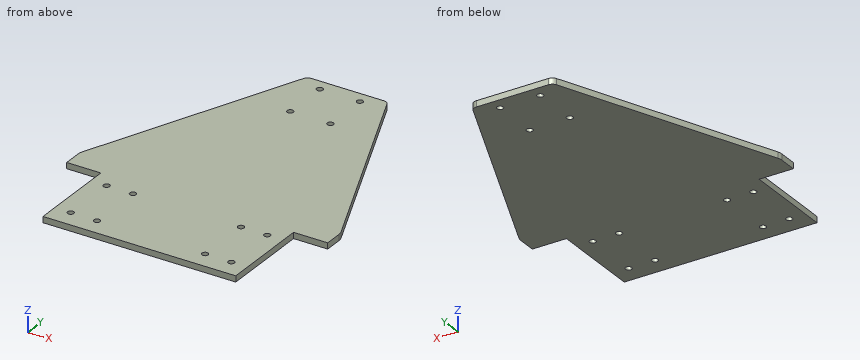
Autodesk Fusion 360 part; units mm, degrees
sketch "Main" plane through (0, 0, 0) normal (0, 0, 1) x (1, 0, 0)
  line L0 (0, 55) -> (45, 162)
  line L1 (45, 162) -> (85, 162)
  line L2 (85, 162) -> (130, 55)
  line L3 (113, 0) -> (17, 0)
  line L4 (65, 0) -> (65, 162) construction
  line L5 (0, 55) -> (0, 45)
  line L6 (0, 45) -> (17, 45)
  line L7 (17, 45) -> (17, 0)
  line L8 (130, 55) -> (130, 45)
  line L9 (130, 45) -> (113, 45)
  line L10 (113, 45) -> (113, 0)
  dimension "d2" = 162
  dimension "d6" = 55
  dimension "d9" = 40
  dimension "d45" = 130
  dimension "d47" = 17
  dimension "d48" = 17
  dimension "d49" = 10
  dimension "d50" = 10
extrude "Extrude1" add sketch "Main" along normal blind 3
sketch "Head Tube Holes" plane through (0, 0, 3) normal (0, 0, 1) x (-1, 0, 0)
  line L0 (-17, 0) -> (-113, 0)
  line L1 (-130, -55) -> (-85, -162)
  line L2 (-85, -162) -> (-45, -162)
  line L3 (-45, -162) -> (0, -55)
  circle A0 centre (-55, -156) radius 1.55
  line L4 (-65, -162) -> (-65, 0) construction
  circle A1 centre (-75, -156) radius 1.55
  circle A2 centre (-55, -133) radius 1.55
  circle A3 centre (-75, -133) radius 1.55
  line L5 (0, -55) -> (0, -45)
  line L6 (0, -45) -> (-17, -45)
  line L7 (-17, -45) -> (-17, 0)
  line L8 (-113, 0) -> (-113, -45)
  line L9 (-113, -45) -> (-130, -45)
  line L10 (-130, -45) -> (-130, -55)
  dimension "d19" = 3.1
  dimension "d20" = 6
  dimension "d21" = 10
  dimension "d24" = -20
  dimension "d25" = 23
extrude "Extrude2" cut sketch "Head Tube Holes" against normal up to surface (3 mm away) contours A0 | A1 | A2 | A3
sketch "Motor Box Holes" plane through (0, 0, 3) normal (0, 0, 1) x (-1, 0, 0)
  circle A0 centre (-75, -156) radius 1.55
  circle A1 centre (-55, -156) radius 1.55
  circle A2 centre (-75, -133) radius 1.55
  circle A3 centre (-55, -133) radius 1.55
  line L0 (-17, 0) -> (-113, 0)
  line L1 (-17, -37) -> (-113, -37) construction
  circle A4 centre (-25, -37) radius 1.55
  circle A5 centre (-38.1, -37) radius 1.55
  circle A6 centre (-25, -9.1) radius 1.55
  circle A7 centre (-38.1, -9.1) radius 1.55
  circle A8 centre (-105, -37) radius 1.55
  circle A9 centre (-91.9, -37) radius 1.55
  circle A10 centre (-105, -9.1) radius 1.55
  circle A11 centre (-91.9, -9.1) radius 1.55
  line L2 (-17, -45) -> (-17, 0)
  line L3 (-113, 0) -> (-113, -45)
  dimension "d30" = 3.1
  dimension "d32" = 37
  dimension "d35" = -13.1
  dimension "d36" = 27.9
  dimension "d37" = 3.1
  dimension "d40" = 13.1
  dimension "d41" = 27.9
  dimension "d53" = 8
  dimension "d54" = 8
extrude "Extrude3" cut sketch "Motor Box Holes" against normal through all contours A4 | A5 | A6 | A7 | A8 | A9 | A10 | A11
fillet "Fillet5" radius 3 2 edges at (45, 162, 1.5) (85, 162, 1.5)
fillet "Fillet6" radius 6 2 edges at (0, 55, 1.5) (130, 55, 1.5)
Work out the finished part from the listing and answer in its coordinate system (mm). Round coordinates to 2 decimals unless told otherwise and drop trailing zeros. Write each loop counter-clockwise with the first axis right and the second up, starting at its lowest first coordinate (ties: lowest second). Pieces come first, ordered by that corner, then holes. Notation, with made-up numbers: (7, 80.5) - (38, 80.5) arc R25 ccw to (38, 115.5) - close; hole circle Ø8 at (70, -31.75). An arc over 180 degrees is marked (long way). Answer in a Markdown table with one row per item. Add a question column.
1. Given pin 1 (3 mm diameter, centred on x = 105, y = 9.1, fed in from +Z); pin 2 (0.9 mm diameter, centred on y = 31, z = 2, fed in from -X); pin 3 (0.9 mm diameter, centred on y = 13.5, z = 2, fed in from +X); pin 4 (1.5 mm diameter, centred on x = 120.5, z = 2, fed in from -Y), each flat-ended and moving along its own axis, determine where each tip first touches the part or whether it passes through.
2. Find the intervals of material crossed by line 1 along Y through (x, z) = (75, 1.85); line 2 along X through (y, z) = (37, 2.05); line 3 along X through (y, z) = (133, 1.35), in increasing order. Write a range as from..to.
3. A cutting plane is placed at A-A, the plane z = 1.4. Count the separate pieces of the cut face and the enclosed holes in it, and give its area (3 significant figures).
4. A cutting plane is placed at B-B, the plane y = 22. Determine the outline of the cut face in (x, z), and give its area (3 significant figures).
5. A cutting plane is placed at C-C, the plane x = 9. Determine the outline of the cut face in (y, z).
Worked out:
| question | item | result |
|---|---|---|
| 1 | pin 1 | through |
| 1 | pin 2 | x = 17 |
| 1 | pin 3 | x = 113 |
| 1 | pin 4 | y = 45 |
| 2 | line 1 | 0..131.45, 134.55..154.45, 157.55..162 |
| 2 | line 2 | 17..23.45, 26.55..36.55, 39.65..90.35, 93.45..103.45, 106.55..113 |
| 2 | line 3 | 32.8..53.45, 56.55..73.45, 76.55..97.2 |
| 3 | separate pieces | 1 |
| 3 | enclosed holes | 12 |
| 3 | area | 14,600 mm^2 |
| 4 | outline | (17, 0) - (113, 0) - (113, 3) - (17, 3) - close |
| 4 | area | 288 mm^2 |
| 5 | outline | (45, 0) - (76.4, 0) - (76.4, 3) - (45, 3) - close |
